Geometry check sheet. Reference: drawing and pictorial views, mm from the part's lowest x, y, z. A direction names the side the tool comes from. Round coordinates to 2 decimals unless told otherwise and drop trailing zeros. Loops run counter-clockwise (first coordinate to the right, second up) from the corner with the lowest first, then second, coordinate; pieces in that order, holes last. Notation, with made-up numbers: (-39, 26.25) - (-30, 26.25) arc R25 ccw to (-30, 57.25) - close; hole circle Ø10 at (69, 16.25). An arc over 180 degrees is marked (long way). Return JSON: item names as keys, results as strings.
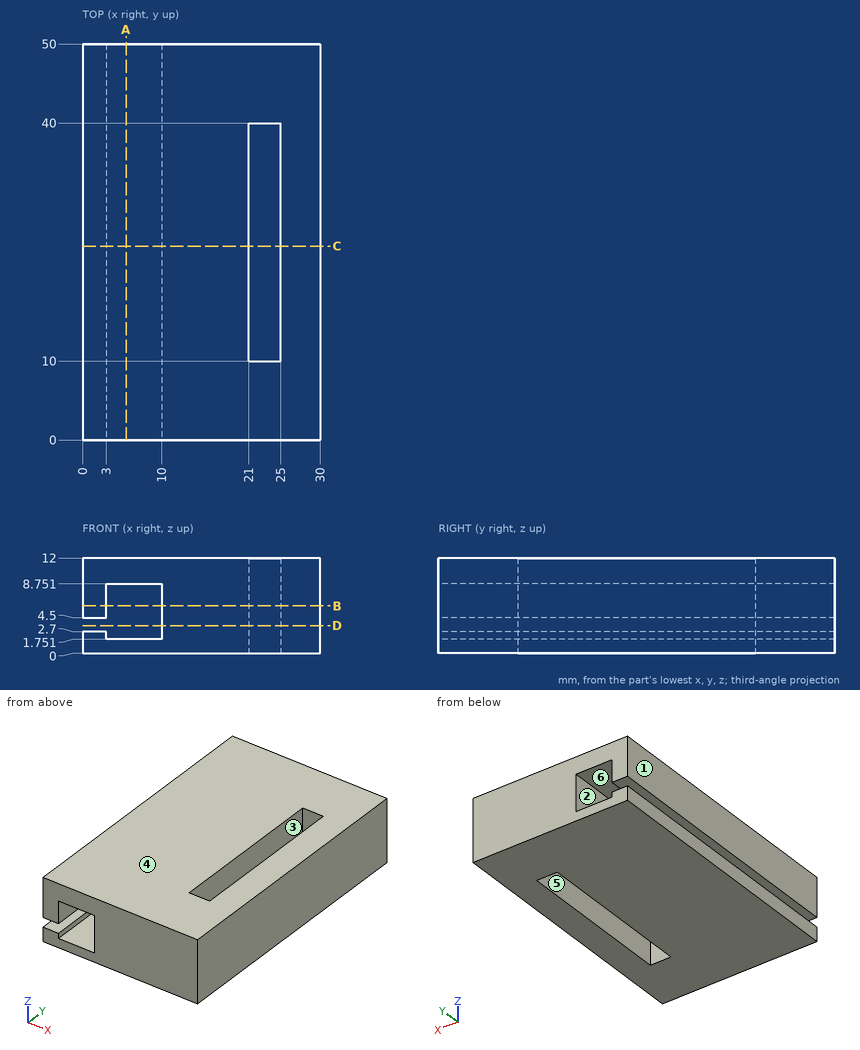
Q1. Sectioned sample at B-B (z = 6). Enter the section's corners in (x, y).
Answer key:
{"outline": "(0, 0) - (3, 0) - (3, 50) - (0, 50) - close; (10, 0) - (30, 0) - (30, 50) - (10, 50) - close; hole (21, 10) - (25, 10) - (25, 40) - (21, 40) - close"}
Q2. Draft check along Z on the marked faces 4, 5 and 6. Enter one of: released by +Z, released by -Z, zero draft, split by the parting line, or undercut.
Answer key:
{"face 4": "released by +Z", "face 5": "zero draft", "face 6": "undercut"}
Q3. Scan lines: probe 1 along X at (y, z) = (32.5, 2); probe 2 along X at (y, z) = (12, 3.5); probe 3 along X at (y, z) = (25, 9.5). Record each from-to range of solid material in increasing order. Write a range as [from, to].
Answer key:
{"probe 1": "x = [0, 3], [10, 21], [25, 30]", "probe 2": "x = [10, 21], [25, 30]", "probe 3": "x = [0, 21], [25, 30]"}
Q4. Sectioned sample at A-A (x = 5.5). Enter the section's corners in (y, z), plus the area to 3 significant figures.
Answer key:
{"outline": "(0, 0) - (50, 0) - (50, 1.75) - (0, 1.75) - close; (0, 8.75) - (50, 8.75) - (50, 12) - (0, 12) - close", "area": "250 mm²"}
Q5. Sectioned sample at D-D (z = 3.5). Enter the section's corners in (x, y).
Answer key:
{"outline": "(10, 0) - (30, 0) - (30, 50) - (10, 50) - close; hole (21, 10) - (25, 10) - (25, 40) - (21, 40) - close"}
Q6. Sectioned sample at C-C (y = 24.5). Enter the section's corners in (x, z), plus the area to 3 significant figures.
Answer key:
{"outline": "(0, 0) - (21, 0) - (21, 12) - (0, 12) - (0, 4.5) - (3, 4.5) - (3, 8.75) - (10, 8.75) - (10, 1.75) - (3, 1.75) - (3, 2.7) - (0, 2.7) - close; (25, 0) - (30, 0) - (30, 12) - (25, 12) - close", "area": "258 mm²"}
Q7. Tool access check on the marked faces 1, 2 and 3. Record the directions out of +Z, -Z, +X, -X, +Y, -Y that give a thin tool (end or side, any length) a straight path to the whole face; none if there is none.
Answer key:
{"face 1": "+Z, -Z, -X, +Y, -Y", "face 2": "+Y, -Y", "face 3": "+Z, -Z"}
